```python
from build123d import *

# Parameters (mm, degrees)
F2_DEPTH = 147.32
F3_DEPTH = 543
F1_R     = 66.04
F4_DEPTH = 147.321


# Not quite as in the source:
# - an extrude ends at something that could not be found from the text; its depth is read off the source's solid


with BuildPart() as f2:
    # F0 (on Right) → F2 (new body)
    with BuildSketch(Plane.YZ):
        Polygon((-227.214354679, -72.635721945), (-227.214354679, -133.595721945), (153.785645321, -133.595721945), (153.785645321, -72.635721945), (59.805645321, -72.635721945), (59.805645321, -6.595721945), (-3.4203693569, -6.595721945), (-97.4624507428, -6.595721945), (-133.234354679, -6.595721945), (-133.234354679, -72.635721945), align=None)
    extrude(amount=F2_DEPTH)

    # F1 (on face) → F3 (cut, through all)
    with BuildSketch(Plane.YZ):
        with BuildLine():
            ThreePointArc((29.3256430177, -6.595721945), (29.3256447452, -6.587001079), (29.325645321, -6.5782802129))
            ThreePointArc((29.325645321, -6.5782802129), (-36.7230755452, 59.4617192113), (-102.7543523758, -6.595721945))
            Line((-102.7543523758, -6.595721945), (-97.4624507428, -6.595721945))
            Line((-97.4624507428, -6.595721945), (-3.4203693569, -6.595721945))
            Line((-3.4203693569, -6.595721945), (29.3256430177, -6.595721945))
        make_face()
    extrude(amount=-F3_DEPTH, mode=Mode.SUBTRACT)

    # F1 (on face) + F2_face (on face) → F4 (cut, through all)
    with BuildSketch(Plane.YZ):
        with Locations((-36.714354679, -6.5782802129)):
            Circle(F1_R)
    with BuildSketch(Plane(origin=(147.32, -36.714354679, -80.6128525046), x_dir=(0, 1, 0), z_dir=(1, 0, 0))):
        Polygon((-190.5, 7.9771305595), (-190.5, -52.9828694405), (190.5, -52.9828694405), (190.5, 7.9771305595), (96.52, 7.9771305595), (96.52, 74.0171305595), (-96.52, 74.0171305595), (-96.52, 7.9771305595), align=None)
    extrude(amount=F4_DEPTH, mode=Mode.SUBTRACT)


solid = f2.part
```
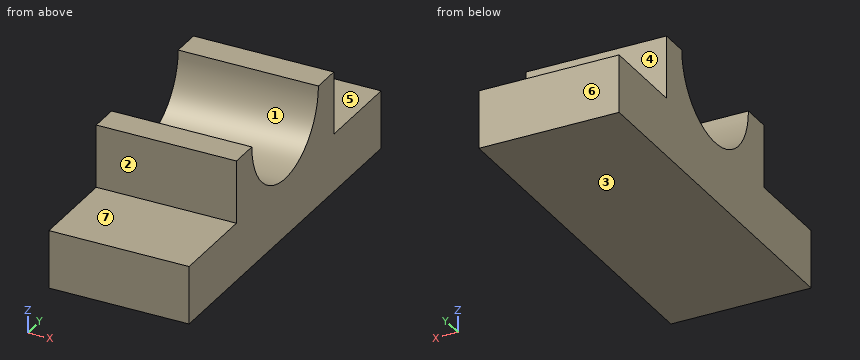
The model under review builds one solid part; all positions refer to its coordinate system, in mm. Face numbers are marked on the shaded views. A direction names the side the tool comes from. Round coordinates to 2 decimals unless told otherwise and drop trailing zeros. Loops run counter-clockwise (first coordinate to the right, second up) from the corner with the lowest first, then second, coordinate; pieces in that order, holes last. Notation, with made-up numbers: (71.5, -39.5) - (119.5, -39.5) arc R22 cw to (119.5, -31.5) - close; hole circle Ø2 at (12, -5.5). An arc over 180 degrees is marked (long way). Use a Markdown table: item, result. Add a question column.
Q1. For probe 1 along Z at (x, y) = (103, 123); probe 2 along Y at (x, z) = (89, -66.5); probe 3 along Y at (x, z) = (97.5, -54), list the stretches that pass through material, from the lowest coordinate up.
Q2. The part is to be moulded in two halves that separate along Y. For the marked faces 1, 2, 3 and 4, say which applies: pulls with the +Y half, pulls with the -Y half, needs draft (parallel to the pull), parting line crosses it, or undercut.
Q3. Add section C-C (y = -81). State the section outline as (x, z) points.
Q4. Add section B-B (z = -28). State the section outline as (x, y) points, plus the area to 3 significant figures.
Q5. Add section D-D (z = -52). State the section outline as (x, y) points, plus the area to 3 significant figures.
Q6. Machinability: for the marked faces 5, 6 and 7, which of the approach directions +Z, -Z, +X, -X, +Y, -Y give a long, thin tool a straight path to every point of the face, cutting with its end or side? Answer none if there is none.
Q7. Insertion check: pin 1 Ø5 at (x, z) = (40.5, -67.5) entering from -Y; pin 2 Ø1 at (x, z) = (69.5, -70.5) entering from +Y. Each pin has a flat end and moves straight along its axis. Give the tip position at first contact, or say it passes through.
Q8. Add section A-A (x = 79). State the section outline as (y, z) points.
Worked answers:
| question | item | result |
|---|---|---|
| 1 | probe 1 | -133.6 to -72.64 |
| 1 | probe 2 | -133.23 to -64.48, -8.95 to 59.81 |
| 1 | probe 3 | -133.23 to -82.68, 9.25 to 59.81 |
| 2 | face 1 | undercut |
| 2 | face 2 | pulls with the -Y half |
| 2 | face 3 | needs draft |
| 2 | face 4 | pulls with the +Y half |
| 3 | outline | (0, -133.6) - (147.32, -133.6) - (147.32, -55.57) - (0, -55.57) - close |
| 4 | outline | (0, -133.23) - (147.32, -133.23) - (147.32, -99.18) - (0, -99.18) - close; (0, 25.75) - (147.32, 25.75) - (147.32, 59.81) - (0, 59.81) - close |
| 4 | area | 10,000 mm² |
| 5 | outline | (0, -133.23) - (147.32, -133.23) - (147.32, -84.65) - (0, -84.65) - close; (0, 11.22) - (147.32, 11.22) - (147.32, 59.81) - (0, 59.81) - close |
| 5 | area | 14,300 mm² |
| 6 | face 5 | +Z, +X, -X, +Y |
| 6 | face 6 | +Z, -Z, +X, -X, +Y |
| 6 | face 7 | +Z, +X, -X, -Y |
| 7 | pin 1 | y = -133.23 |
| 7 | pin 2 | y = 59.81 |
| 8 | outline | (-227.21, -133.6) - (153.79, -133.6) - (153.79, -72.64) - (59.81, -72.64) - (59.81, -6.6) - (29.33, -6.6) arc R66.04 cw to (-102.75, -6.6) - (-133.23, -6.6) - (-133.23, -72.64) - (-227.21, -72.64) - close |
